Check sheet for the modelled part. Datum: model origin and axes. Units: mm. Coordinates: 2 decimals unless noted, no trailing zeros. Order: outer loops, then holes, each group sorted by start corner. A loop starts at its lowest first (then second) coordinate and runs counter-clockwise, first axis right, second up. Notation, with made-up numbers: (36.5, -30.5) -> (64.5, -30.5) arc R23 cw to (64.5, 3.5) -> close; hole circle Ø6 at (-23.75, -32). An arc over 180 degrees is marked (long way). Put each result on its own line as item: value. Start each with the question number.
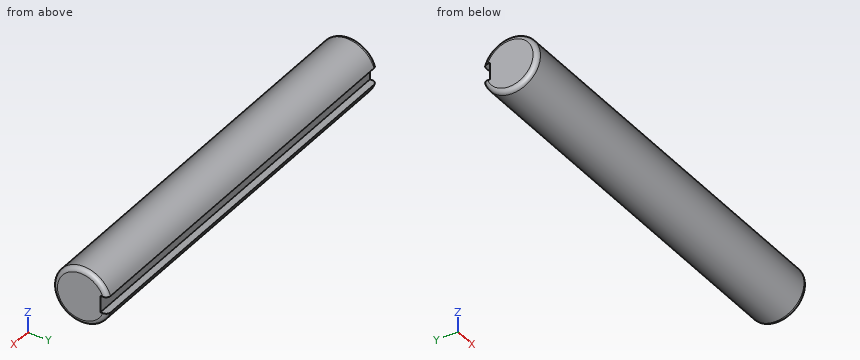
```python
from build123d import *

# Parameters (mm, degrees)
SKETCH1_R          = 7.9375
EXTRUDE1_DEPTH     = 114.3
SKETCH2_W          = 4.7625
SKETCH2_H          = 2.38125
CUT_EXTRUDE1_DEPTH = 115.3
FILLET1_R          = 1.27


with BuildPart() as part:
    # Sketch1 → Extrude1 (new body)
    with BuildSketch(Plane(origin=(0, 0, 0), x_dir=(0, 0, -1), z_dir=(1, 0, 0))):
        Circle(SKETCH1_R)
    extrude(amount=EXTRUDE1_DEPTH)

    # Sketch2 → Cut-Extrude1 (cut, through all)
    with BuildSketch(Plane.ZY):
        with Locations((0, 6.746875)):
            Rectangle(SKETCH2_W, SKETCH2_H)
    extrude(amount=-CUT_EXTRUDE1_DEPTH, mode=Mode.SUBTRACT)

    # Fillet1
    fillet1_edges = [part.edges().sort_by_distance(p)[0] for p in [
        (0, -7.9375, 0),
        (114.3, -7.9375, 0),
    ]]
    fillet(fillet1_edges, radius=FILLET1_R)


solid = part.part
```
1) Sectioned sample at B-B (x = 71.5). Record the boundary of the cut face in (y, z) (1 decimal).
2) Gauge pin test, flat ends, axial feed: pin 1 (2 mm diameter, centred on x = 80.5, y = 6.5, fed in from -Z); pin 2 (2 mm diameter, centred on x = 85, y = 3, fed in from +Z); pin 3 (0.6 mm diameter, centred on x = 41, y = 6.5, fed in from +Z). Record the tip position at first contact, or that the pin passes through.
3) Scan lines: line 1 along Y through (x, z) = (29, -0.5); line 2 along Z through (x, y) = (54, 6); line 3 along Z through (x, y) = (88.5, -0.5). Record each from-to range of solid material in increasing order. Write a range as [from, to].
4) Sectioned sample at A-A (z = 0). Record the boundary of the cut face in (x, y).
Entries:
1. outline: (5.6, -2.4) -> (5.6, 2.4) -> (7.6, 2.4) arc R7.9 ccw (long way) to (7.6, -2.4) -> close
2. pin 1: stops at z = -5.72
2. pin 2: stops at z = 7.68
2. pin 3: stops at z = 4.96
3. line 1: y = [-7.92, 5.56]
3. line 2: z = [-5.2, -2.38], [2.38, 5.2]
3. line 3: z = [-7.92, 7.92]
4. outline: (0, -6.67) arc R1.27 ccw to (1.27, -7.94) -> (113.03, -7.94) arc R1.27 ccw to (114.3, -6.67) -> (114.3, 5.56) -> (0, 5.56) -> close
